from build123d import *

# Parameters (mm, degrees)
BOSS_EXTRUDE1_DEPTH  = 10
M8_CLEARANCE_HOLE4_D = 9
M8_CLEARANCE_HOLE5_D = 9
CIRPATTERN1_COUNT    = 4
CIRPATTERN2_COUNT    = 4


with BuildPart() as part:
    # Sketch1 → Boss-Extrude1 (new body)
    with BuildSketch(Plane(origin=(0, 0, 0), x_dir=(1, 0, 0), z_dir=(0, 1, 0))):
        Polygon((-200, 0), (200, 0), (315.470053838, 200), (-315.470053838, 200), align=None)
    extrude(amount=BOSS_EXTRUDE1_DEPTH)

    # M8 Clearance Hole4 (through all)
    with Locations(Plane(origin=(0, 10, 0), x_dir=(1, 0, 0), z_dir=(0, 1, 0))):
        with Locations((-170.675979174, 51.703708686)):
            m8_clearance_hole4 = Hole(M8_CLEARANCE_HOLE4_D / 2)

    # M8 Clearance Hole5 (through all)
    with Locations(Plane(origin=(0, 10, 0), x_dir=(1, 0, 0), z_dir=(0, 1, 0))):
        with Locations((170.675979174, 51.703708686)):
            m8_clearance_hole5 = Hole(M8_CLEARANCE_HOLE5_D / 2)

    # CirPattern1: M8 Clearance Hole5 ×4 about axis
    cirpattern1_axis = Axis((157.735026919, 0, -100), (0, 1, 0))
    for i in range(1, CIRPATTERN1_COUNT):
        add(m8_clearance_hole5.rotate(cirpattern1_axis, i * 360 / CIRPATTERN1_COUNT), mode=Mode.SUBTRACT)

    # CirPattern2: M8 Clearance Hole4 ×4 about axis
    cirpattern2_axis = Axis((-157.735026919, 0, -100), (0, 1, 0))
    for i in range(1, CIRPATTERN2_COUNT):
        add(m8_clearance_hole4.rotate(cirpattern2_axis, i * 360 / CIRPATTERN2_COUNT), mode=Mode.SUBTRACT)


solid = part.part
Read the model definition and answer for the solid it produces. Units are mm, in the model's axes. Round coordinates to 2 decimals unless told otherwise and drop trailing zeros. Write each loop counter-clockwise with the first axis right and the second up, starting at its lowest first coordinate (ties: lowest second). Pieces come first, ordered by that corner, then holes.
1. The part is cut by section B-B, the plane x = 235. Determine the outline of the cut face in (y, z), then the cut area to 3 significant figures.
2. Straight lines are drawn through the part: L1, parallel to X at y = 1.5, z = -89.5; L2, parallel to X at y = 4.5, z = -90.5; L3, parallel to Z at x = 204, y = 8.25. For each, find the intervals that lie inside material, in ascending order.
3. Given pin 1 Ø3 at (y, z) = (7, -67) entering from -X, flat-ended and moving along its own axis, determine where the tip first touches the part or whether it passes through.
4. The part is cut by section A-A, the plane y = 4.25. State how many separate pieces and enclosed holes the cut face has, then the cut area to 3 significant figures.
5. The part is cut by section C-C, the plane z = -28.5. Determine the outline of the cut face in (x, y), then the cut area to 3 significant figures.
Values:
1. outline: (0, -200) - (10, -200) - (10, -60.62) - (0, -60.62) - close
1. area: 1,390 mm2
2. L1: x = -251.67 to -113.22, -105.66 to 105.66, 113.22 to 251.67
2. L2: x = -252.25 to -112.34, -106.54 to 106.54, 112.34 to 252.25
2. L3: z = -200 to -116.96, -108.93 to -6.93
3. pin 1: stops at x = -239.55
4. separate pieces: 1
4. enclosed holes: 8
4. area: 103,000 mm2
5. outline: (-216.45, 0) - (216.45, 0) - (216.45, 10) - (-216.45, 10) - close
5. area: 4,330 mm2
